The listing builds one solid part. Answer for the finished solid, in the listing's coordinates (mm). Round coordinates to 2 decimals unless told otherwise and drop trailing zeros. Write each question's results on one line, items separated by ' | '. Start each with the question number.
(1) Determine the mould class of faces 1 (the face through (0, -1, 0)), 2 (the face through (1.9, -0.6, 9.6)) for opening direction X: released by +X, released by -X, zero draft, split by the parting line, or undercut.
(2) Straight lines are drawn through the part: probe 1 along X at (y, z) = (-2.75, 9.5); probe 2 along Y at (x, z) = (-4.5, 7.5); probe 3 along X at (y, z) = (-6, 4.75). For each, find the intervals that lie inside material, in ascending order.
(3) Flat-ended cylindrical pins translate along their axes: pin 1 (6 mm diameter, centred on x = 0.5, z = 7, fed in from +Y); pin 2 (5 mm diameter, centred on x = 7.5, z = 7, fed in from +Y); pin 3 (4 mm diameter, centred on x = -2, y = 2.5, fed in from +Z). Find the tip coordinate at first contact, or state that the pin passes through.
```python
from build123d import *

# Parameters (mm, degrees)
F1_ANGLE = 180
F3_R     = 5.5
F3_R_2   = 5
F4_DEPTH = 16
F5_R     = 2
F6_DEPTH = 5


with BuildPart() as f1:
    # F0 (on Top) → F1 (revolve)
    with BuildSketch(Plane.XY):
        with BuildLine():
            Line((0, 8.77414), (0, 8.586648))
            Line((0, 8.586648), (0, -11.213352))
            Line((0, -11.213352), (0, -11.22586))
            Line((0, -11.22586), (0.5, -11.22586))
            ThreePointArc((0.5, -11.22586), (10.5, -1.22586), (0.5, 8.77414))
            Line((0.5, 8.77414), (0, 8.77414))
        make_face()
    revolve(axis=Axis((0, -1.313352, 0), (0, -1, 0)), revolution_arc=F1_ANGLE)

    # F3 (on offset) → F4 (cut)
    with BuildSketch(Plane.XY.offset(25)):
        with Locations((0, -1.22586)):
            Circle(F3_R)
        with Locations((0, -1.22586)):
            Circle(F3_R_2, mode=Mode.SUBTRACT)
    extrude(amount=-F4_DEPTH, mode=Mode.SUBTRACT)

    # F5 (on face) → F6 (cut)
    with BuildSketch(Plane.XY.offset(9)):
        with Locations((0, -1.22586)):
            Circle(F5_R)
    extrude(amount=F6_DEPTH, mode=Mode.SUBTRACT)


solid = f1.part
```
Checked values:
1) face 1: zero draft | face 2: undercut
2) probe 1: x = -4.19 to -1.29, 1.29 to 4.19 | probe 2: y = -6.88 to 4.43 | probe 3: x = -7.98 to 7.98
3) pin 1: stops at y = 8.13 | pin 2: stops at y = 5.65 | pin 3: stops at z = 10.25
